Could you check a few things on this model? Use its own coordinates, in mm. Round coordinates to 2 decimals unless told otherwise and drop trailing zeros. Return JSON: item names as keys, results as strings. Group by question number.
```python
from build123d import *

# Parameters (mm, degrees)
F0_R     = 15.875
F1_DEPTH = 6.35
F2_R     = 2.0955
F3_DEPTH = 6.35
F7_R     = 1.5875


with BuildPart() as f1:
    # F0 (on Front) → F1 (new body)
    with BuildSketch(Plane.XZ):
        Circle(F0_R)
    extrude(amount=F1_DEPTH)

    # F2 (on face) → F3 (cut)
    with BuildSketch(Plane.XZ.offset(6.35)):
        Circle(F2_R)
    extrude(amount=-F3_DEPTH, mode=Mode.SUBTRACT)

    # F4 (on Right) → F6 (revolve, cut)
    with BuildSketch(Plane.YZ):
        with BuildLine():
            Line((-1.778, 15.875), (-4.572, 15.875))
            Line((-4.572, 15.875), (-3.397973, 13.598685))
            ThreePointArc((-3.397973, 13.598685), (-3.175, 13.462803), (-2.952027, 13.598685))
            Line((-2.952027, 13.598685), (-1.778, 15.875))
        make_face()
    revolve(axis=Axis((0, -3.17588, 0), (0, -1, 0)), mode=Mode.SUBTRACT)

    # F7
    f7_edges = [f1.edges().sort_by_distance(p)[0] for p in [
        (-11.22532, -4.572, -11.22532),
        (-11.22532, -1.778, -11.22532),
    ]]
    fillet(f7_edges, radius=F7_R)


solid = f1.part
```
1. We'd pull the mould along Z, two halves only. Please class faces 1 (the face through (2, -3.22, 0.63)), 2 (the face through (14.664, -5.939, -6.08)), 3 (the face through (3, -6.35, 0)): +Z half, -Z half, draft (parallel to the pull), parting line (faces both ways), or undercut.
2. I need wall thicknesses on probe 1 along Z at (x, y) = (0, -4.75); probe 2 along Y at (x, z) = (-13.5, 0.5); probe 3 along Z at (x, y) = (0, -4.25). Which ranges of each line are inside material? Lowest first, please.
3. I'm going to push flat-ended pins straight in: pin 1 Ø4 at (x, z) = (-5.5, -1.5) entering from +Y; pin 2 Ø3 at (y, z) = (-4.5, -2) entering from +X; pin 3 Ø1.5 at (y, z) = (-3.5, -8.5) entering from -X. Where does each tip first touch, or does it pass through?
Geometry results:
{
 "1": {"face 1": "undercut", "face 2": "parting line", "face 3": "draft"},
 "2": {"probe 1": "-15.66 to -2.1, 2.1 to 15.66", "probe 2": "-6.35 to -3.32, -3.03 to 0", "probe 3": "-15.21 to -2.1, 2.1 to 15.21"},
 "3": {"pin 1": "y = 0", "pin 2": "x = 15.85", "pin 3": "x = -12.71"}
}
